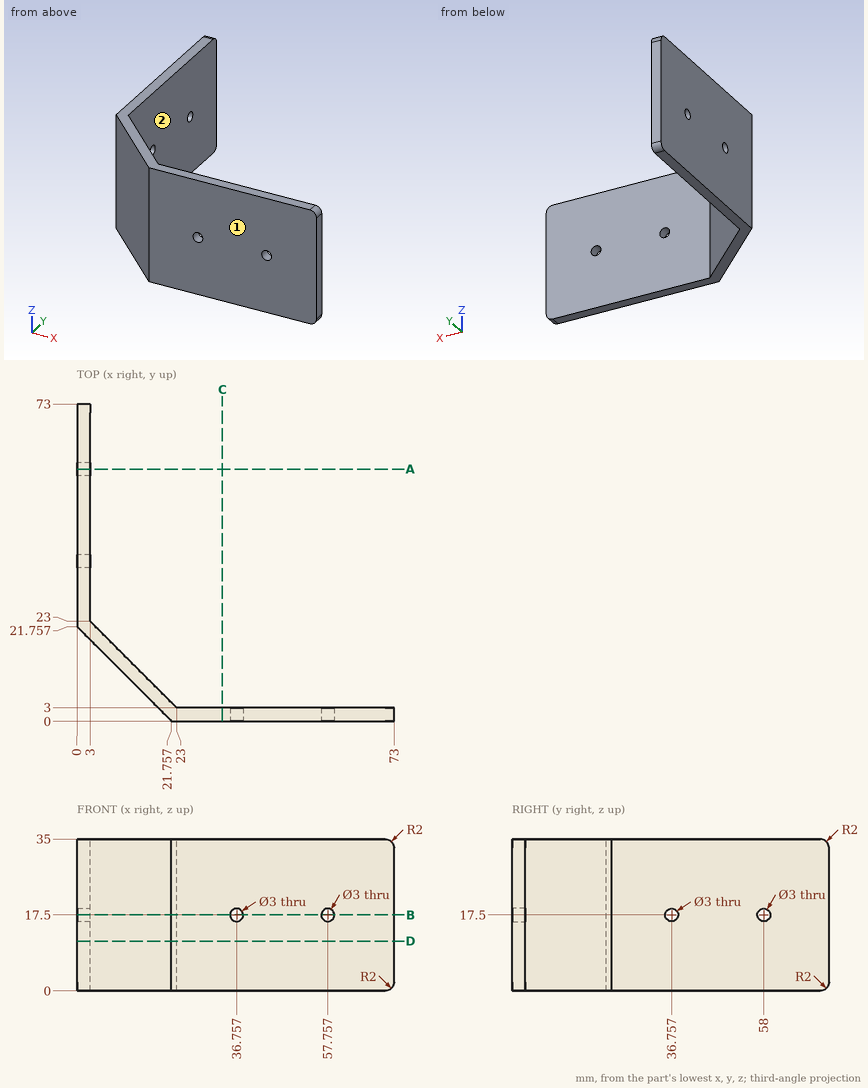
Design review of the part shown in the three views and the two pictorial views. Dimensions are in mm from the part's minimum x, y and z. A direction names the side the tool comes from. Give positions to 0.01 mm unless a question says otherwise; leave off trailing zeros. Loops run counter-clockwise (first coordinate to the right, second up) from the corner with the lowest first, then second, coordinate; pieces in that order, holes last. Notation, with made-up numbers: (-27, 44) -> (17, 44) arc R14 ccw to (17, 51) -> close; hole circle Ø2 at (14.25, 3.5). An arc over 180 degrees is marked (long way). One line per question, with ' | ' between items.
1) For the marked faces 1 and 2, list the 3-axis set-ups (+Z, -Z, +X, -X, +Y, -Y) from which the entire face can be reached by the end or side of a thin tool; tool diameter is ignored.
Resolved:
face 1: +Z, -Z, +X, -X, -Y | face 2: +Z, -Z, +X, +Y
2) To check wall thickness, follow probe 1 along X at (y, z) = (1.7, 17.5); probe 2 along X at (y, z) = (0.9, 17.5); probe 3 along Y at (x, z) = (0.7, 17.5). State the ranges of each line that lie inside material, in increasing order.
Resolved:
probe 1: x = 20.06 to 35.26, 38.26 to 56.26, 59.26 to 73 | probe 2: x = 20.86 to 35.26, 38.26 to 56.26, 59.26 to 73 | probe 3: y = 21.06 to 35.26, 38.26 to 56.5, 59.5 to 73
3) We need section C-C (x = 33.5). Write out the cut boundary in (y, z), plus the area to 3 significant figures.
Resolved:
outline: (0, 0) -> (3, 0) -> (3, 35) -> (0, 35) -> close | area: 105 mm2
4) We need section D-D (z = 11.5). Write out the cut boundary in (x, y).
Resolved:
outline: (0, 21.76) -> (21.76, 0) -> (73, 0) -> (73, 3) -> (23, 3) -> (3, 23) -> (3, 73) -> (0, 73) -> close
5) We need section A-A (y = 58). Write out the cut boundary in (x, z).
Resolved:
outline: (0, 0) -> (3, 0) -> (3, 16) -> (0, 16) -> close; (0, 19) -> (3, 19) -> (3, 35) -> (0, 35) -> close
6) Insertion check: pin 1 Ø10.5 at (y, z) = (40.5, 10.5) entering from +X; pin 2 Ø8 at (x, z) = (16.5, 7) entering from +Y; pin 3 Ø4 at (x, z) = (57.76, 17.5) entering from +Y; pin 4 Ø1.8 at (y, z) = (36.76, 17.5) entering from +X. Each pin has a flat end and moves straight along its axis. Give the tip position at first contact, or say it passes through.
Resolved:
pin 1: stops at x = 3 | pin 2: stops at y = 13.5 | pin 3: stops at y = 3 | pin 4: passes through
7) We need section B-B (z = 17.5). Write out the cut boundary in (x, y).
Resolved:
outline: (0, 21.76) -> (21.76, 0) -> (35.26, 0) -> (35.26, 3) -> (23, 3) -> (3, 23) -> (3, 35.26) -> (0, 35.26) -> close; (0, 38.26) -> (3, 38.26) -> (3, 56.5) -> (0, 56.5) -> close; (0, 59.5) -> (3, 59.5) -> (3, 73) -> (0, 73) -> close; (38.26, 0) -> (56.26, 0) -> (56.26, 3) -> (38.26, 3) -> close; (59.26, 0) -> (73, 0) -> (73, 3) -> (59.26, 3) -> close
